Job drawing, mm, ordinate dimensions from the low corner. One solid piece. A direction names the side the tool comes from. Give positions to 0.01 mm unless a question says otherwise; leave off trailing zeros. Order: outer loops, then holes, each group sorted by start corner. A loop starts at its lowest first (then second) coordinate and runs counter-clockwise, first axis right, second up. Notation, with made-up numbers: (-3.5, 19.5) - (52.5, 19.5) arc R24 cw to (52.5, 42.5) - close; hole circle Ø7 at (16, -30). An arc over 180 degrees is marked (long way). Use one line per item in the form item = value. Start each with the question number.
1. Drill centre lines: line 1 (Z direction, x = 12.5, y = 3.5) (1 decimal); line 2 (X direction, y = 15.75, z = 19.5); line 3 (Y direction, x = 16, z = 13). Where is each one in solid material? Low to high.
2. Band-saw the part on C-C, the plane z = 19. List the corners of the cut face in (x, y), plus the area to 3 significant figures.
3. Band-saw the part on A-A, the plane x = 11.75. List the corners of the cut face in (y, z) (1 decimal).
4. Band-saw the part on D-D, the plane x = 19. List the corners of the cut face in (y, z) (1 decimal).
5. Pin check, flat tips, straight feed: P1, Ø4, axis at x = 13, z = 16, coming from the +Y side; P2, Ø5.5, axis at x = 6.5, z = 11.5, coming from the -Y side; P3, Ø12, axis at x = 15.5, z = 10.5, coming from the +Y side (1 decimal). Stop position of each tip, or through.
6. Tool access for the marked faces 4, 5 and 6: list every direction of +Z, -Z, +X, -X, +Y, -Y with a clear straight run to the whole face (end or side of a thin tool).
7. Pull direction X, two halves, no side cores. Call the marked faces 1, 2 and 3: +X half, -X half, draft (parallel to the pull), parting line (faces both ways), or undercut.
8. Band-saw the part on B-B, the plane y = 16.5. State how many separate pieces and enclosed holes the cut face has, plus the area to 3 significant figures.
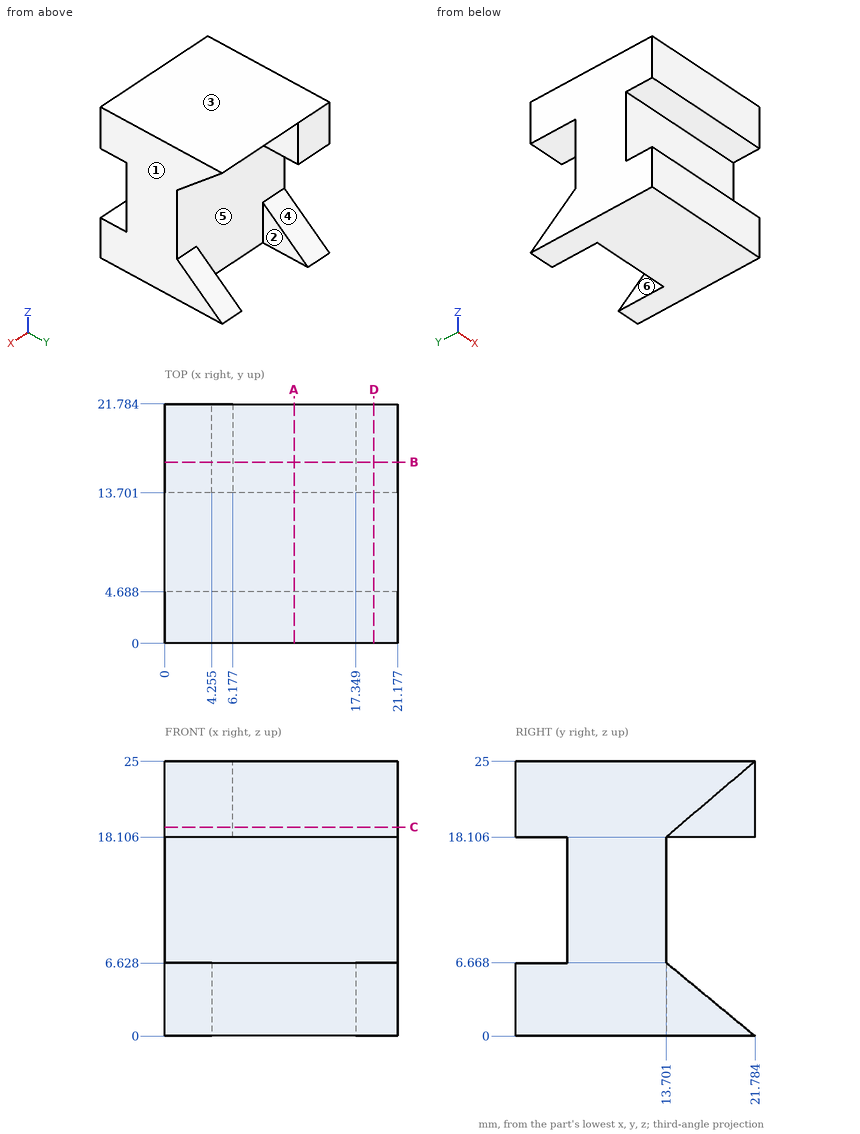
From the geometry:
q1.line_1 = 0 to 6.6, 18.1 to 25
q1.line_2 = 0 to 6.18
q1.line_3 = 4.69 to 13.7
q2.outline = (0, 0) - (21.18, 0) - (21.18, 14.75) - (6.18, 14.75) - (6.18, 21.78) - (0, 21.78) - close
q2.area = 356 mm²
q3.outline = (0, 0) - (13.7, 0) - (13.7, 18.1) - (21.8, 25) - (0, 25) - (0, 18.1) - (4.7, 18.1) - (4.7, 6.6) - (0, 6.6) - close
q4.outline = (0, 0) - (21.8, 0) - (13.7, 6.7) - (13.7, 18.1) - (21.8, 25) - (0, 25) - (0, 18.1) - (4.7, 18.1) - (4.7, 6.6) - (0, 6.6) - close
q5.P1 = 13.7
q5.P2 = 4.69
q5.P3 = 16
q6.face_4 = +X, -X, +Y
q6.face_5 = +Y
q6.face_6 = -Z, +Y
q7.face_1 = +X half
q7.face_2 = undercut
q7.face_3 = draft
q8.separate_pieces = 3
q8.enclosed_holes = 0
q8.area = 145 mm²
